For this review, take the finished solid that the model builds, in its own axes (mm). Round coordinates to 2 decimals unless told otherwise and drop trailing zeros. Write each loop counter-clockwise with the first axis right and the second up, starting at its lowest first coordinate (ties: lowest second). Pieces come first, ordered by that corner, then holes. Notation, with made-up numbers: M 2.5,9.25 L 38.5,9.25 A28 ccw 38.5,28.25 Z; hole C 4.25,-23.75 d9. An arc over 180 degrees is marked long. Write each question's results on one line, items separated by ' | '. Start each with the question number.
```python
from build123d import *

# Parameters (mm, degrees)
SKETCH1_R           = 1.5
SKETCH1_R_2         = 5
SKETCH1_R_3         = 7.55
SKETCH1_R_4         = 2
SKETCH1_R_5         = 1.625
BOSS_EXTRUDE1_DEPTH = 5


with BuildPart() as part:
    # Sketch1 → Boss-Extrude1 (new body)
    with BuildSketch(Plane.XZ):
        with BuildLine():
            Line((-184.068782704, -199.369837197), (-184.068782704, -249.965787275))
            ThreePointArc((-184.068782704, -249.965787275), (-181.139850516, -257.036855087), (-174.068782704, -259.965787275))
            Line((-174.068782704, -259.965787275), (25.931217296, -259.965787275))
            ThreePointArc((25.931217296, -259.965787275), (33.002285108, -257.036855087), (35.931217296, -249.965787275))
            Line((35.931217296, -249.965787275), (35.931217296, -199.369837197))
            ThreePointArc((35.931217296, -199.369837197), (35.013998456, -196.483507693), (32.598858094, -194.65613651))
            ThreePointArc((32.598858094, -194.65613651), (30.55061758, -193.655934533), (28.782088358, -192.21788113))
            ThreePointArc((28.782088358, -192.21788113), (-11.089192992, -94.369837197), (28.782088358, 3.478206737))
            ThreePointArc((28.782088358, 3.478206737), (30.55061758, 4.916260139), (32.598858094, 5.916462116))
            ThreePointArc((32.598858094, 5.916462116), (34.466751202, 14.165696709), (26.217516609, 12.297803601))
            ThreePointArc((26.217516609, 12.297803601), (25.217314632, 10.249563087), (23.77926123, 8.481033865))
            ThreePointArc((23.77926123, 8.481033865), (-74.068782704, -31.390247486), (-171.916826637, 8.481033865))
            ThreePointArc((-171.916826637, 8.481033865), (-173.35488004, 10.249563087), (-174.355082017, 12.297803601))
            ThreePointArc((-174.355082017, 12.297803601), (-182.60431661, 14.165696709), (-180.736423502, 5.916462116))
            ThreePointArc((-180.736423502, 5.916462116), (-178.688182988, 4.916260139), (-176.919653766, 3.478206737))
            ThreePointArc((-176.919653766, 3.478206737), (-137.048372415, -94.369837197), (-176.919653766, -192.21788113))
            ThreePointArc((-176.919653766, -192.21788113), (-178.688182988, -193.655934533), (-180.736423502, -194.65613651))
            ThreePointArc((-180.736423502, -194.65613651), (-183.151563863, -196.483507693), (-184.068782704, -199.369837197))
        make_face()
        with Locations(Location((-179.068782704, -199.369837197, 0), (0, 0, 90))):
            Circle(SKETCH1_R, mode=Mode.SUBTRACT)
        with Locations(Location((-179.068782704, 10.630162803, 0), (0, 0, 90))):
            Circle(SKETCH1_R, mode=Mode.SUBTRACT)
        with Locations(Location((30.931217296, 10.630162803, 0), (0, 0, 90))):
            Circle(SKETCH1_R, mode=Mode.SUBTRACT)
        with Locations(Location((30.931217296, -199.369837197, 0), (0, 0, 90))):
            Circle(SKETCH1_R, mode=Mode.SUBTRACT)
        with Locations(Location((-74.068782704, -239.369837197, 0), (0, 0, 90))):
            Circle(SKETCH1_R_2, mode=Mode.SUBTRACT)
        with Locations(Location((5.931217296, -239.369837197, 0), (0, 0, 90))):
            Circle(SKETCH1_R_3, mode=Mode.SUBTRACT)
        with Locations(Location((-154.068782704, -239.369837197, 0), (0, 0, 90))):
            Circle(SKETCH1_R_3, mode=Mode.SUBTRACT)
        with Locations(Location((-154.068782704, -251.369837197, 0), (0, 0, 90))):
            Circle(SKETCH1_R_4, mode=Mode.SUBTRACT)
        with Locations(Location((-142.068782704, -239.369837197, 0), (0, 0, 90))):
            Circle(SKETCH1_R_4, mode=Mode.SUBTRACT)
        with Locations(Location((-154.068782704, -227.369837197, 0), (0, 0, 90))):
            Circle(SKETCH1_R_4, mode=Mode.SUBTRACT)
        with Locations(Location((-166.068782704, -239.369837197, 0), (0, 0, 90))):
            Circle(SKETCH1_R_4, mode=Mode.SUBTRACT)
        with Locations(Location((5.931217296, -251.369837197, 0), (0, 0, 90))):
            Circle(SKETCH1_R_4, mode=Mode.SUBTRACT)
        with Locations(Location((-6.068782704, -239.369837197, 0), (0, 0, 90))):
            Circle(SKETCH1_R_4, mode=Mode.SUBTRACT)
        with Locations(Location((5.931217296, -227.369837197, 0), (0, 0, 90))):
            Circle(SKETCH1_R_4, mode=Mode.SUBTRACT)
        with Locations(Location((17.931217296, -239.369837197, 0), (0, 0, 90))):
            Circle(SKETCH1_R_4, mode=Mode.SUBTRACT)
        with Locations(Location((-73.929921751, -247.368631958, 0), (0, 0, 90))):
            Circle(SKETCH1_R_5, mode=Mode.SUBTRACT)
        with Locations(Location((-66.069987942, -239.230976244, 0), (0, 0, 90))):
            Circle(SKETCH1_R_5, mode=Mode.SUBTRACT)
        with Locations(Location((-74.207643657, -231.371042435, 0), (0, 0, 90))):
            Circle(SKETCH1_R_5, mode=Mode.SUBTRACT)
        with Locations(Location((-82.067577465, -239.50869815, 0), (0, 0, 90))):
            Circle(SKETCH1_R_5, mode=Mode.SUBTRACT)
        with Locations(Location((-130.068782704, -219.369837197, 0), (0, 0, 90))):
            Circle(SKETCH1_R_4, mode=Mode.SUBTRACT)
        with Locations(Location((-98.068782704, -219.369837197, 0), (0, 0, 90))):
            Circle(SKETCH1_R_4, mode=Mode.SUBTRACT)
        with Locations(Location((-18.068782704, -219.369837197, 0), (0, 0, 90))):
            Circle(SKETCH1_R_4, mode=Mode.SUBTRACT)
        with Locations(Location((-50.068782704, -219.369837197, 0), (0, 0, 90))):
            Circle(SKETCH1_R_4, mode=Mode.SUBTRACT)
        with BuildLine():
            Line((-135.716591192, -209.257050985), (-12.420974216, -209.257050985))
            ThreePointArc((-12.420974216, -209.257050985), (-3.488029353, -203.751769673), (-4.390759374, -193.297550202))
            ThreePointArc((-4.390759374, -193.297550202), (-33.466178067, -128.862078617), (-33.094357447, -58.171402287))
            ThreePointArc((-33.094357447, -58.171402287), (-34.169669225, -54.470723718), (-37.870347793, -53.39541194))
            ThreePointArc((-37.870347793, -53.39541194), (-74.068782704, -57.390247486), (-110.267217614, -53.39541194))
            ThreePointArc((-110.267217614, -53.39541194), (-113.967896183, -54.470723718), (-115.04320796, -58.171402287))
            ThreePointArc((-115.04320796, -58.171402287), (-114.671387341, -128.862078617), (-143.746806034, -193.297550202))
            ThreePointArc((-143.746806034, -193.297550202), (-144.649536054, -203.751769673), (-135.716591192, -209.257050985))
        make_face(mode=Mode.SUBTRACT)
    extrude(amount=-BOSS_EXTRUDE1_DEPTH)


solid = part.part
```
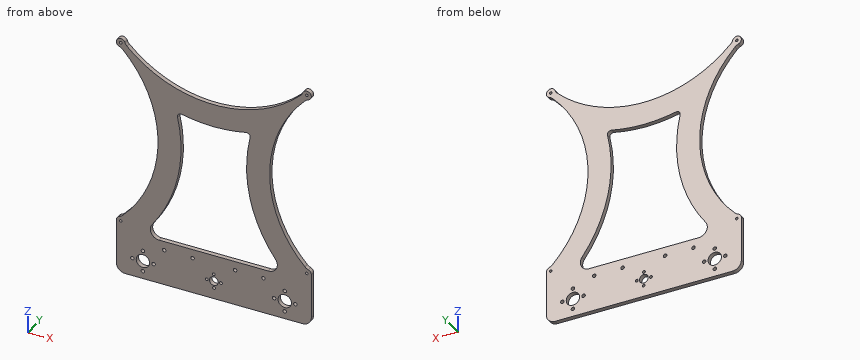
Item 1: We need section C-C on y = 4. State how many separate pieces and enclosed holes the cut face has, then the cut area to 3 significant figures.
Item 2: We need section B-B on x = -26. State the section outline as (y, z) points.
Item 3: We need section D-D on z = -47. State the section outline as (x, y) points.
Item 4: For probe 1 along Z at (x, y) = (-18, 0.4); probe 2 along X at (y, z) = (1.1, -237); probe 3 along Z at (x, y) = (-126, 2.8), list the stretches that pass through material, from the lowest coordinate up.
Item 5: We need section A-A on z = -18. State the section outline as (x, y) points, then the cut area to 3 significant figures.
Item 6: Insertion check: P1, Ø1, axis at y = 1, z = -141.5, coming from the -X side. The pin has a flat end and moves straight along its axis. Give the tip position at first contact, or say it passes through.
Numbers:
1) separate pieces: 1 | enclosed holes: 24 | area: 24,900 mm^2
2) outline: M 0,-259.97 L 5,-259.97 L 5,-209.26 L 0,-209.26 Z; M 0,-154.02 L 5,-154.02 L 5,-22.88 L 0,-22.88 Z
3) outline: M -145.31,0 L -2.83,0 L -2.83,5 L -145.31,5 Z
4) probe 1: z = -259.97 to -221.37, -217.37 to -209.26, -171.66 to -19.67 | probe 2: x = -184.07 to -161.24, -146.9 to -78.47, -69.67 to -1.24, 13.1 to 35.93 | probe 3: z = -259.97 to -209.26, -163.22 to -21.4
5) outline: M -159.71,0 L -133.82,0 L -133.82,5 L -159.71,5 Z; M -14.32,0 L 11.58,0 L 11.58,5 L -14.32,5 Z | area: 259 mm^2
6) P1: stops at x = -145.4
